Could you check a few things on this model? Use its own coordinates, in mm. A direction names the side the tool comes from. Round coordinates to 2 decimals unless told otherwise and drop trailing zeros. Loops run counter-clockwise (first coordinate to the right, second up) from the corner with the lowest first, then second, coordinate; pieces in that order, holes last.
from build123d import *

# Parameters (mm, degrees)
SKETCH_1_R                       = 3.5
EXTRUDE_1_DEPTH                  = 45
HOLE_WIZARD_M4_1_D               = 3.3
HOLE_WIZARD_M4_1_DEPTH           = 12.1
HOLE_WIZARD_M4_1_TIP             = 0.991420021
HOLE_WIZARD_M4_1_ON_FACE_2_D     = 3.3
HOLE_WIZARD_M4_1_ON_FACE_2_DEPTH = 12.1
HOLE_WIZARD_M4_1_ON_FACE_2_TIP   = 0.991420021
CHAMFER_1_SIZE                   = 0.5


with BuildPart() as part:
    # 草图1 → 拉伸1 (new, symmetric)
    with BuildSketch(Plane.XY):
        with Locations(Location((0, 0, 0), (0, 0, 180))):
            Circle(SKETCH_1_R)
    extrude(amount=EXTRUDE_1_DEPTH, both=True)

    # M4 螺纹孔1
    with Locations(Plane.XY.offset(45)):
        with Locations((0, 0)):
            Hole(HOLE_WIZARD_M4_1_D / 2, depth=HOLE_WIZARD_M4_1_DEPTH)
            with Locations((0, 0, -(HOLE_WIZARD_M4_1_DEPTH + HOLE_WIZARD_M4_1_TIP / 2))):  # 118° drill point
                Cone(0, HOLE_WIZARD_M4_1_D / 2, HOLE_WIZARD_M4_1_TIP, mode=Mode.SUBTRACT)

    # M4 螺纹孔1 on face 2
    with Locations(Plane(origin=(0, 0, -45), x_dir=(-1, 0, 0), z_dir=(0, 0, -1))):
        with Locations((0, 0)):
            Hole(HOLE_WIZARD_M4_1_ON_FACE_2_D / 2, depth=HOLE_WIZARD_M4_1_ON_FACE_2_DEPTH)
            with Locations((0, 0, -(HOLE_WIZARD_M4_1_ON_FACE_2_DEPTH + HOLE_WIZARD_M4_1_ON_FACE_2_TIP / 2))):  # 118° drill point
                Cone(0, HOLE_WIZARD_M4_1_ON_FACE_2_D / 2, HOLE_WIZARD_M4_1_ON_FACE_2_TIP, mode=Mode.SUBTRACT)

    # 倒角1
    chamfer_1_edges = [part.edges().sort_by_distance(p)[0] for p in [
        (3.5, 0, -45),
        (3.5, 0, 45),
        (-1.65, 0, -45),
        (1.65, 0, 45),
    ]]
    chamfer(chamfer_1_edges, length=CHAMFER_1_SIZE)


solid = part.part
Item 1: If we section it at A-A, the plane z = -15: Please give me the cut outline in (x, y).
Results list:
outline: circle Ø7 at (0, 0)
Item 2: Will these pins go through, and if not, where does the flat tip stop? pin 1 (4 mm diameter, centred on y = 0.5, z = -18, fed in from +X); pin 2 (1.5 mm diameter, centred on x = 1, z = -33.5, fed in from -Y); pin 3 (4 mm diameter, centred on x = 0, y = 0, fed in from +Z).
Results list:
pin 1: stops at x = 3.5
pin 2: stops at y = -3.49
pin 3: stops at z = 44.85
Item 3: We'd pull the mould along Y, two halves only. Please class faces 4 (the flat face through (-1.3, 2, 45)), 5 (the conical face through (-0.1, -0.3, 32.1)), 6 (the cylindrical face through (-3.233, 1.341, 0.623)): released by +Y, released by -Y, zero draft, split by the parting line, or undercut.
Results list:
face 4: zero draft
face 5: undercut
face 6: split by the parting line
Item 4: For faces 1 (the flat face through (-1.3, 2, -45)), 2 (the cylindrical face through (1.216, 1.115, 38.619)), 3 (the cylindrical face through (-1.216, 1.115, -38.619)), which set-ups out of +Z, -Z, +X, -X, +Y, -Y let a thin tool reach every point of the face, with its end or its side?
Results list:
face 1: -Z, +X, -X, +Y, -Y
face 2: +Z
face 3: -Z
Item 5: If I drill on line 1 along Y through (x, z) = (0, -35.25); line 2 along X through (y, z) = (-1.25, 35.5); line 3 along Z through (x, y) = (-1.25, -1), over which ranges is the centre line in solid material (lowest first)?
Results list:
line 1: y = -3.5 to -1.65, 1.65 to 3.5
line 2: x = -3.27 to -1.08, 1.08 to 3.27
line 3: z = -32.87 to 32.87
